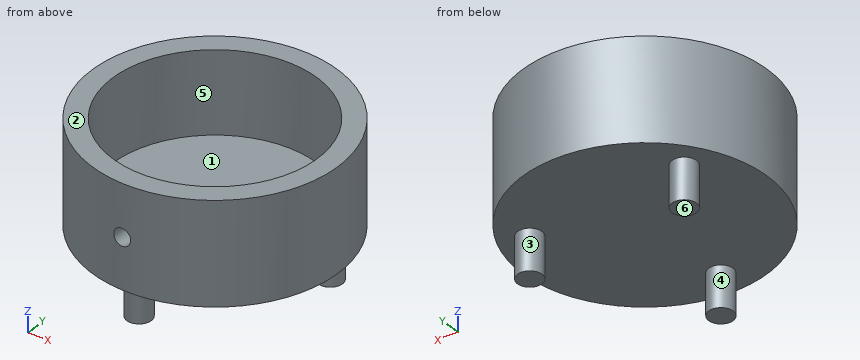
```python
from build123d import *

# Parameters (mm, degrees)
F0_R     = 30
F0_R_2   = 25
F1_DEPTH = 25
F2_R     = 30
F3_DEPTH = 5
F4_R     = 3
F5_DEPTH = 10
F9_D     = 4.2
F9_DEPTH = 12


with BuildPart() as f1:
    # F0 (on Top) → F1 (new body)
    with BuildSketch(Plane.XY):
        Circle(F0_R)
        Circle(F0_R_2, mode=Mode.SUBTRACT)
    extrude(amount=F1_DEPTH)

    # F2 (on Top) → F3 (join)
    with BuildSketch(Plane.XY):
        Circle(F2_R)
    extrude(amount=F3_DEPTH)

    # F4 (on face) → F5 (join)
    with BuildSketch(Plane.XY):
        with Locations((-1.107393, -23.067445)):
            Circle(F4_R)
        with Locations((-19.423297, 12.492753)):
            Circle(F4_R)
        with Locations((20.53069, 10.574692)):
            Circle(F4_R)
    extrude(amount=-F5_DEPTH)

    # F9
    with Locations(Plane.XZ.offset(30)):
        with Locations((0, 12.374512)):
            Hole(F9_D / 2, depth=F9_DEPTH)


solid = f1.part
```
Part model, mm, in its own coordinate system. Face numbers are marked on the shaded views. A direction names the side the tool comes from. Give positions to 0.01 mm unless a question says otherwise; leave off trailing zeros. Write each loop counter-clockwise with the first axis right and the second up, starting at its lowest first coordinate (ties: lowest second). Pieces come first, ordered by that corner, then holes. Notation, with made-up numbers: M 26,-1 L 72,-1 A25 ccw 72,29 Z; hole C 39,74 d1. An arc over 180 degrees is marked long. Use CSV: the item, a comma, the result in double quotes.
Item 1: Drill centre lines: probe 1 along X at (y, z) = (0.5, 18) (3 decimals); probe 2 along Z at (x, y) = (0, -28.3); probe 3 along Y at (x, z) = (0, 15). Where is each one in solid material? Low to high.
Taken from the geometry:
probe 1,"x = -29.996 to -24.995, 24.995 to 29.996"
probe 2,"z = 0 to 10.27, 14.47 to 25"
probe 3,"y = -30 to -25, 25 to 30"
Item 2: Slice it at A-A on y = 0. Write the cut outline in (x, z).
Taken from the geometry:
outline,"M -30,0 L 30,0 L 30,25 L 25,25 L 25,5 L -25,5 L -25,25 L -30,25 Z"
Item 3: Pin check, flat tips, straight feed: P1, Ø25, axis at x = 0.5, y = 6, coming from the +Z side; P2, Ø4, axis at x = -17, z = 3.5, coming from the +Y side; P3, Ø4, axis at y = -2.5, z = 17.5, coming from the -X side. Stop position of each tip, or through.
Taken from the geometry:
P1,"stops at z = 5"
P2,"stops at y = 25.98"
P3,"stops at x = -30"
Item 4: Pull direction X, two halves, no side cores. Call the marked faces 4, 5 and 6: +X half, -X half, draft (parallel to the pull), parting line (faces both ways), or undercut.
Taken from the geometry:
face 4,"parting line"
face 5,"undercut"
face 6,"draft"
Item 5: Slice it at C-C on z = 19. Write the cut outline in (x, y), plus the area to 3 significant figures.
Taken from the geometry:
outline,"C 0,0 d60; hole C 0,0 d50"
area,"864 mm²"
Item 6: Slice it at B-B on x = 0. Write the cut outline in (y, z).
Taken from the geometry:
outline,"M -30,0 L -25.86,0 L -25.86,-10 L -20.28,-10 L -20.28,0 L 30,0 L 30,25 L 25,25 L 25,5 L -25,5 L -25,10.27 L -30,10.27 Z; M -30,14.47 L -25,14.47 L -25,25 L -30,25 Z"
Item 7: Which spindle directions (+Z, -Z, +X, -X, +Y, -Y) get a long thin tool onto all of the face, cutting with end or side? Do the marked faces 1, 2 and 3. Say none if no direction does.
Taken from the geometry:
face 1,"+Z"
face 2,"+Z, +X, -X, +Y, -Y"
face 3,"-Z"
Item 8: Slice it at D-D on x = -24. Write the cut outline in (y, z).
Taken from the geometry:
outline,"M -18,0 L 18,0 L 18,25 L 7,25 L 7,5 L -7,5 L -7,25 L -18,25 Z"
